from build123d import *

# Parameters (mm, degrees)
SKETCH1_R           = 60.325
SKETCH1_R_2         = 53.975
BOSS_EXTRUDE1_DEPTH = 50.8
BOSS_EXTRUDE2_START = -1.351993
SKETCH2_R           = 12.7
BOSS_EXTRUDE2_DEPTH = 26.751993
SKETCH3_R           = 3.175
CUT_EXTRUDE1_DEPTH  = 50.8
FILLET1_R           = 1.27


with BuildPart() as part:
    # Sketch1 → Boss-Extrude1 (new body)
    with BuildSketch(Plane(origin=(0, 0, 0), x_dir=(1, 0, 0), z_dir=(0, 1, 0))):
        with Locations(Location((0, 0, 0), (0, 0, 270))):
            Circle(SKETCH1_R)
        with Locations(Location((0, 0, 0), (0, 0, 270))):
            Circle(SKETCH1_R_2, mode=Mode.SUBTRACT)
    extrude(amount=BOSS_EXTRUDE1_DEPTH)

    # Sketch2 → Boss-Extrude2 (add)
    with BuildSketch(Plane.ZY.offset(60.325).offset(BOSS_EXTRUDE2_START)):
        with Locations(Location((0, 25.4, 0), (0, 0, 180))):
            Circle(SKETCH2_R)
    boss_extrude2 = extrude(amount=BOSS_EXTRUDE2_DEPTH)

    # Sketch3 → Cut-Extrude1 (cut)
    with BuildSketch(Plane.ZY.offset(85.725)):
        with Locations((0, 25.4)):
            Circle(SKETCH3_R)
    cut_extrude1 = extrude(amount=-CUT_EXTRUDE1_DEPTH, mode=Mode.SUBTRACT)

    # Mirror1: Boss-Extrude2, Cut-Extrude1 across plane
    add(boss_extrude2.mirror(Plane(origin=(0, 0, 0), x_dir=(0, 0, 1), z_dir=(1, 0, 0))))
    add(cut_extrude1.mirror(Plane(origin=(0, 0, 0), x_dir=(0, 0, 1), z_dir=(1, 0, 0))), mode=Mode.SUBTRACT)

    # Fillet1
    fillet1_edges = [part.edges().sort_by_distance(p)[0] for p in [
        (-85.725, 25.4, 12.7),
        (-85.725, 25.4, -3.175),
        (85.725, 25.4, 12.7),
        (85.725, 25.4, -3.175),
    ]]
    fillet(fillet1_edges, radius=FILLET1_R)


solid = part.part
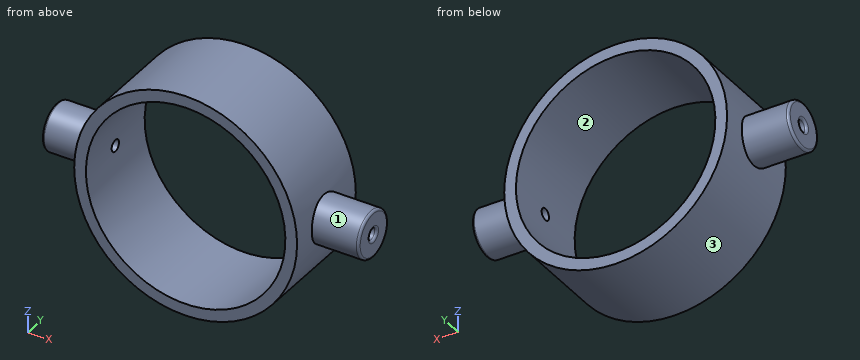
Source: CAD feature listing. Evaluate the final solid. Frame: model axes, mm. Face numbers are marked on the shaded views. Coordinates: 2 decimals unless noted, no trailing zeros. Order: outer loops, then holes, each group sorted by start corner. A loop starts at its lowest first (then second) coordinate and runs counter-clockwise, first axis right, second up. Notation, with made-up numbers: M -19.75,11.25 L 8.25,11.25 A23 cw 8.25,35.25 Z; hole C 4,-23 d2. An arc over 180 degrees is marked long. Write each question's results on one line, items separated by ' | '. Start each with the question number.
Item 1: Cut plane B-B (z = 0). Count the separate pieces of the cut face and the enclosed holes in it, and give its area (3 significant figures).
Item 2: Cut plane D-D (z = -17). Return loops of the section in (x, y).
Item 3: Draft query along X for the marked faces 1, 2 and 3. Return one class per face: pulls with the +X half, pulls with the -X half, needs draft (parallel to the pull), parting line crosses it, or undercut.
Item 4: First-contact query: pin 1 Ø1 at (y, z) = (22, 21) entering from -X; pin 2 Ø6 at (y, z) = (26, -18) entering from +X; pin 3 Ø8 at (x, y) = (10, 41) entering from -Z. Flat tips, straight axial feed; report the tip coordinate or a pass-through.
Item 5: Cut plane A-A (x = 0). Return loops of the section in (y, z) (3 decimals), and give its area (3 significant figures).
Item 6: Cut plane C-C (y = 25.4). Return loops of the section in (x, z) (3 decimals), and give its area (3 significant figures).
Item 7: Line query: probe 1 along Z at (x, y) = (76, 25.4) (3 decimals); probe 2 along Y at (x, z) = (-61, 0) (3 decimals); probe 3 along X at (y, z) = (18, 0) (3 decimals). Output: solid intervals per line, ascending.
Checked values:
1) separate pieces: 4 | enclosed holes: 0 | area: 1,530 mm2
2) outline: M -57.88,0 L -51.23,0 L -51.23,50.8 L -57.88,50.8 Z; M 51.23,0 L 57.88,0 L 57.88,50.8 L 51.23,50.8 Z
3) face 1: needs draft | face 2: undercut | face 3: parting line crosses it
4) pin 1: stops at x = -56.73 | pin 2: stops at x = 58.43 | pin 3: stops at z = -60.03
5) outline: M 0,-60.325 L 50.8,-60.325 L 50.8,-53.975 L 0,-53.975 Z; M 0,53.975 L 50.8,53.975 L 50.8,60.325 L 0,60.325 Z | area: 645 mm2
6) outline: M -85.725,-11.43 A1.27 ccw -84.455,-12.7 L -58.973,-12.7 A60.325 ccw 58.973,-12.7 L 84.455,-12.7 A1.27 ccw 85.725,-11.43 L 85.725,-4.445 A1.27 ccw 84.455,-3.175 L 53.882,-3.175 A53.975 cw -53.882,-3.175 L -84.455,-3.175 A1.27 ccw -85.725,-4.445 Z; M -85.725,4.445 A1.27 ccw -84.455,3.175 L -53.882,3.175 A53.975 cw 53.882,3.175 L 84.455,3.175 A1.27 ccw 85.725,4.445 L 85.725,11.43 A1.27 ccw 84.455,12.7 L 58.973,12.7 A60.325 ccw -58.973,12.7 L -84.455,12.7 A1.27 ccw -85.725,11.43 Z | area: 3,190 mm2
7) probe 1: z = -12.7 to -3.175, 3.175 to 12.7 | probe 2: y = 12.7 to 22.225, 28.575 to 38.1 | probe 3: x = -85.725 to -53.975, 53.975 to 85.725
